```python
from build123d import *

# Parameters (mm, degrees)
SKETCH1_W           = 150
SKETCH1_H           = 125
BOSS_EXTRUDE1_DEPTH = 47.5
SHELL1_T            = -2.5
SKETCH2_R           = 1
SKETCH2_W           = 10
SKETCH2_H           = 10
CUT_EXTRUDE1_DEPTH  = 2.5


with BuildPart() as part:
    # Sketch1 → Boss-Extrude1 (new body)
    with BuildSketch(Plane(origin=(0, 0, 0), x_dir=(1, 0, 0), z_dir=(0, 1, 0))):
        Rectangle(SKETCH1_W, SKETCH1_H)
    extrude(amount=BOSS_EXTRUDE1_DEPTH)

    # Shell1
    shell1_openings = [part.faces().sort_by_distance(p)[0] for p in [
        (0, 47.5, 0),
        (0, 0, 0),
    ]]
    offset(amount=SHELL1_T, openings=shell1_openings, kind=Kind.INTERSECTION)

    # Sketch2 → Cut-Extrude1 (cut)
    with BuildSketch(Plane.XY.offset(62.5)):
        with Locations((-10.5, 12)):
            Circle(SKETCH2_R)
        with Locations((-10.5, 24.5)):
            Circle(SKETCH2_R)
        with Locations((10.5, 12)):
            Circle(SKETCH2_R)
        with Locations((10.5, 24.5)):
            Circle(SKETCH2_R)
        with Locations((0, 24.5)):
            Rectangle(SKETCH2_W, SKETCH2_H)
    extrude(amount=-CUT_EXTRUDE1_DEPTH, mode=Mode.SUBTRACT)


solid = part.part
```
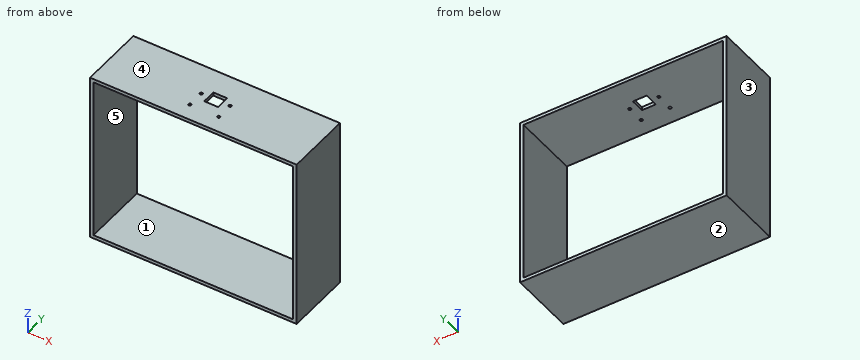
Geometry: final body of the model. Coordinates: model frame, mm. Face numbers are marked on the shaded views. A direction names the side the tool comes from. Round coordinates to 2 decimals unless told otherwise and drop trailing zeros. Order: outer loops, then holes, each group sorted by start corner. A loop starts at its lowest first (then second) coordinate and runs counter-clockwise, first axis right, second up. Notation, with made-up numbers: (79.5, 40.25) -> (120.5, 40.25) arc R14 cw to (120.5, 64.25) -> close; hole circle Ø1 at (-31, 16.25). An arc over 180 degrees is marked (long way). Use one line per item in the form item = value.
(1) Ray query, probe 1 along Y at (x, z) = (10.5, 61.7); probe 2 along X at (y, z) = (23, -36); probe 3 along Z at (x, y) = (-38, 43). Return the intervals inside material, ascending. Write a range as [from, to].
Results list:
probe_1 = [0, 11], [13, 23.5], [25.5, 47.5]
probe_2 = [-75, -72.5], [72.5, 75]
probe_3 = [-62.5, -60], [60, 62.5]
(2) Section C-C on z = -23.5. Return loops of the section in (x, y), and give its area (4 significant figures).
Results list:
outline = (-75, 0) -> (-72.5, 0) -> (-72.5, 47.5) -> (-75, 47.5) -> close; (72.5, 0) -> (75, 0) -> (75, 47.5) -> (72.5, 47.5) -> close
area = 237.5 mm^2
(3) Section A-A on y = 35.5. Return loops of the section in (x, z).
Results list:
outline = (-75, -62.5) -> (75, -62.5) -> (75, 62.5) -> (-75, 62.5) -> close; hole (-72.5, -60) -> (72.5, -60) -> (72.5, 60) -> (-72.5, 60) -> close
(4) Section B-B on x = -61.5. Return loops of the section in (y, z), and give its area (4 significant figures).
Results list:
outline = (0, -62.5) -> (47.5, -62.5) -> (47.5, -60) -> (0, -60) -> close; (0, 60) -> (47.5, 60) -> (47.5, 62.5) -> (0, 62.5) -> close
area = 237.5 mm^2
(5) Draft query along X for the marked faces 3, 4 and 5. Return one class per face: pulls with the +X half, pulls with the -X half, needs draft (parallel to the pull), parting line crosses it, or undercut.
Results list:
face_3 = pulls with the -X half
face_4 = needs draft
face_5 = undercut
(6) Access query for the marked faces 1 and 2. Directions: +Z, -Z, +X, -X, +Y, -Y. A direction counts if a zero-diameter tool reaches every point of the face in a straight line with its end or side. Return the directions, or none.
Results list:
face_1 = +Y, -Y
face_2 = -Z, +X, -X, +Y, -Y
(7) Section D-D on y = 27.5. Return loops of the section in (x, z).
Results list:
outline = (-75, -62.5) -> (75, -62.5) -> (75, 62.5) -> (5, 62.5) -> (5, 60) -> (72.5, 60) -> (72.5, -60) -> (-72.5, -60) -> (-72.5, 60) -> (-5, 60) -> (-5, 62.5) -> (-75, 62.5) -> close
